Geometry: final body of the model. Coordinates: model frame, mm. Coordinates: 2 decimals unless noted, no trailing zeros. Write each loop counter-clockwise with the first axis right and the second up, starting at its lowest first coordinate (ties: lowest second). Pieces come first, ordered by that corner, then holes. Notation, with made-up numbers: (38.25, 51.25) -> (62.25, 51.25) arc R33 cw to (62.25, 83.25) -> close; hole circle Ø10 at (87.5, 44). An arc over 180 degrees is marked (long way). Answer as a JSON object with one key per item and string values. Group by question number.
```python
from build123d import *

# Parameters (mm, degrees)
F0_W     = 67
F0_H     = 20
F1_DEPTH = 45
F2_R     = 3
F4_DEPTH = 5.6
F5_DEPTH = 5.7
F6_W     = 52.390475
F6_H     = 5.804801
F7_DEPTH = 2.2
F6_W_2   = 10.85727
F6_H_2   = 2.118381
F8_DEPTH = 1.3


with BuildPart() as f1:
    # F0 (on Front) → F1 (new body, symmetric)
    with BuildSketch(Plane.XZ):
        Rectangle(F0_W, F0_H)
    extrude(amount=F1_DEPTH, both=True)

    # F2
    f2_edges = [f1.edges().sort_by_distance(p)[0] for p in [
        (-33.5, 0, 10),
        (-33.5, 0, -10),
        (33.5, 0, 10),
        (33.5, 0, -10),
    ]]
    fillet(f2_edges, radius=F2_R)

    # F3 (on face) → F4 (join)
    with BuildSketch(Plane.XZ.offset(45)):
        with BuildLine():
            ThreePointArc((-10.025558, 0), (-12.40529, 2.379732), (-14.785022, 0))
            Line((-14.785022, 0), (-10.025558, 0))
        make_face()
        with BuildLine():
            ThreePointArc((14.566558, 0), (12.115266, 2.451292), (9.663974, 0))
            Line((9.663974, 0), (14.566558, 0))
        make_face()
        with BuildLine():
            Line((14.566558, 0), (9.663974, 0))
            ThreePointArc((9.663974, 0), (12.115266, -2.451292), (14.566558, 0))
        make_face()
        with BuildLine():
            Line((-10.025558, 0), (-14.785022, 0))
            ThreePointArc((-14.785022, 0), (-12.40529, -2.379732), (-10.025558, 0))
        make_face()
    extrude(amount=F4_DEPTH)

    # F3 (on face) → F5 (join)
    with BuildSketch(Plane.XZ.offset(45)):
        with BuildLine():
            ThreePointArc((-10.025558, 0), (-12.40529, 2.379732), (-14.785022, 0))
            Line((-14.785022, 0), (-10.025558, 0))
        make_face()
        with BuildLine():
            ThreePointArc((14.566558, 0), (12.115266, 2.451292), (9.663974, 0))
            Line((9.663974, 0), (14.566558, 0))
        make_face()
        with BuildLine():
            Line((14.566558, 0), (9.663974, 0))
            ThreePointArc((9.663974, 0), (12.115266, -2.451292), (14.566558, 0))
        make_face()
        with BuildLine():
            Line((-10.025558, 0), (-14.785022, 0))
            ThreePointArc((-14.785022, 0), (-12.40529, -2.379732), (-10.025558, 0))
        make_face()
    extrude(amount=F5_DEPTH)

    # F6 (on face) → F7 (join)
    with BuildSketch(Plane(origin=(0, 45, 0), x_dir=(-1, 0, 0), z_dir=(0, 1, 0))):
        with Locations((1.547624, -1.486943)):
            Rectangle(F6_W, F6_H)
    extrude(amount=F7_DEPTH)

    # F6 (on face) → F8 (join)
    with BuildSketch(Plane(origin=(0, 45, 0), x_dir=(-1, 0, 0), z_dir=(0, 1, 0))):
        with Locations((13.856874, 4.369838)):
            Rectangle(F6_W_2, F6_H_2)
    extrude(amount=F8_DEPTH)


solid = f1.part
```
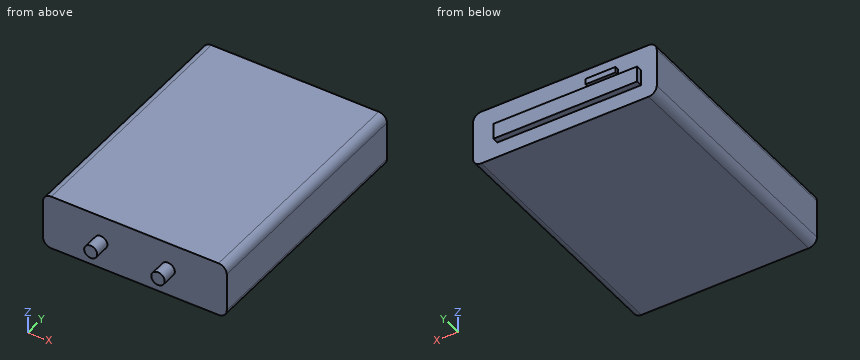
Item 1: Section A-A on x = 17. Output: boundary loops of the cut face in (y, z).
Item 2: Section C-C on x = -13.5. Output: boundary loops of the cut face in (y, z).
Item 3: Ray query, L1, parallel to Y at x = -8, z = -1.25; L2, parallel to Y at x = 0.5, z = -8.5; L3, parallel to Z at x = -31, y = 26. Return the intervals inside material, ascending. Write a range as [from, to].
Item 4: Contact query for flat-ended pins moving along their axis: pin 1 (10 mm diameter, centred on x = 2, z = -2.5, fed in from -Y); pin 2 (1.1 mm diameter, centred on x = -11.5, z = 4.5, fed in from +Y); pin 3 (2.5 mm diameter, centred on y = 46, z = -2.5, fed in from +X); pin 4 (1.8 mm diameter, centred on y = 46, z = -3, fed in from -X). Output: stop coordinate, or through.
Item 5: Section B-B on z = 0. Output: boundary loops of the cut face in (x, y), then the cut area to 3 significant figures.
Answer sheet:
{
 "1": {"outline": "(-45, -10) -> (45, -10) -> (45, -4.39) -> (47.2, -4.39) -> (47.2, 1.42) -> (45, 1.42) -> (45, 10) -> (-45, 10) -> close"},
 "2": {"outline": "(-50.7, -2.11) -> (-45, -2.11) -> (-45, -10) -> (45, -10) -> (45, -4.39) -> (47.2, -4.39) -> (47.2, 1.42) -> (45, 1.42) -> (45, 3.31) -> (46.3, 3.31) -> (46.3, 5.43) -> (45, 5.43) -> (45, 10) -> (-45, 10) -> (-45, 2.11) -> (-50.7, 2.11) -> close"},
 "3": {"L1": "y = [-45, 47.2]", "L2": "y = [-45, 45]", "L3": "z = [-9.96, 9.96]"},
 "4": {"pin 1": "stops at y = -45", "pin 2": "stops at y = 46.3", "pin 3": "stops at x = 33.5", "pin 4": "stops at x = -27.74"},
 "5": {"outline": "(-33.5, -45) -> (-14.79, -45) -> (-14.79, -50.7) -> (-10.03, -50.7) -> (-10.03, -45) -> (9.66, -45) -> (9.66, -50.7) -> (14.57, -50.7) -> (14.57, -45) -> (33.5, -45) -> (33.5, 45) -> (24.65, 45) -> (24.65, 47.2) -> (-27.74, 47.2) -> (-27.74, 45) -> (-33.5, 45) -> close", "area": "6,200 mm^2"}
}
